Could you check a few things on this model? Use its own coordinates, in mm. A direction names the side the tool comes from. Coordinates: 2 decimals unless noted, no trailing zeros. Order: outer loops, then holes, each group sorted by start corner. A loop starts at its lowest first (then second) coordinate and runs counter-clockwise, first axis right, second up. Notation, with made-up numbers: (12.5, 37.5) -> (68.5, 37.5) arc R16 ccw to (68.5, 65.5) -> close; hole circle Ø2 at (-6, -39.75). An arc over 180 degrees is marked (long way). Return JSON: item names as keys, results as strings. Group by question number.
from build123d import *

# Parameters (mm, degrees)
F0_R     = 17.5
F1_DEPTH = 15
F2_R     = 4.5
F3_DEPTH = 3
F4_R     = 1.6
F5_DEPTH = 5


with BuildPart() as f1:
    # F0 (on Right) → F1 (new body)
    with BuildSketch(Plane.YZ):
        Circle(F0_R)
    extrude(amount=F1_DEPTH)

    # F2 (on face) → F3 (join)
    with BuildSketch(Plane.YZ.offset(15)):
        Circle(F2_R)
    extrude(amount=F3_DEPTH)

    # F4 (on face) → F5 (cut)
    with BuildSketch(Plane.YZ.offset(18)):
        Circle(F4_R)
    extrude(amount=-F5_DEPTH, mode=Mode.SUBTRACT)


solid = f1.part
Q1. I want a section at C-C on x = 9.25. Please give me the cut outline in (y, z), and give its area (3 significant figures).
Q2. On a 3-axis mill with a long thin cutter (end or side, diameter ignored), from which of +Z, -Z, +X, -X, +Y, -Y can I reach the whole of each face in a straight line? I mean faces 5 (the flat face through (0, 0, 0)), 6 (the cylindrical face through (16.48, -0.59, 4.46)). Say none if no direction works.
Q3. I want a section at D-D on y = 12.5. Please give me the cut outline in (x, z).
Q4. I'm going to push flat-ended pins straight in: pin 1 Ø1.5 at (y, z) = (-6.5, 4.5) entering from +X; pin 2 Ø8 at (x, z) = (14.5, 11) entering from +Y; pin 3 Ø2 at (x, z) = (10.5, 8) entering from -Y. Where does each tip first touch, or does it pass through?
Q5. I want a section at A-A on z = 0. Please give me the cut outline in (x, y), and give its area (3 significant figures).
Q6. I need wall thicknesses on line 1 along Z through (x, y) = (14.65, 0); line 2 along X through (y, z) = (0.5, 14); line 3 along Z through (x, y) = (16.95, 0). Which ranges of each line are inside material? Lowest first, please. Write a range as from..to.
Q7. We'd pull the mould along Z, two halves only. Please class faces 1 (the cylindrical face through (7.395, -13.887, -10.648)), 2 (the flat face through (18, 0, -2)), 3 (the flat face through (13, 0, 0)), 4 (the cylindrical face through (15.54, -1.27, -0.97)): pulls with the +Z half, pulls with the -Z half, needs draft (parallel to the pull), parting line crosses it, or undercut.
Response values:
{
 "1": {"outline": "circle Ø35 at (0, 0)", "area": "962 mm²"},
 "2": {"face 5": "+Z, -Z, -X, +Y, -Y", "face 6": "+X"},
 "3": {"outline": "(0, -12.25) -> (15, -12.25) -> (15, 12.25) -> (0, 12.25) -> close"},
 "4": {"pin 1": "stops at x = 15", "pin 2": "stops at y = 16.04", "pin 3": "stops at y = -16.04"},
 "5": {"outline": "(0, -17.5) -> (15, -17.5) -> (15, -4.5) -> (18, -4.5) -> (18, -1.6) -> (13, -1.6) -> (13, 1.6) -> (18, 1.6) -> (18, 4.5) -> (15, 4.5) -> (15, 17.5) -> (0, 17.5) -> close", "area": "536 mm²"},
 "6": {"line 1": "z = -17.5..-1.6, 1.6..17.5", "line 2": "x = 0..15", "line 3": "z = -4.5..-1.6, 1.6..4.5"},
 "7": {"face 1": "parting line crosses it", "face 2": "needs draft", "face 3": "undercut", "face 4": "undercut"}
}
